from build123d import *

# Parameters (mm, degrees)
F1_DEPTH  = 76.2
F2_R      = 12.7
F3_DEPTH  = 76.201
F5_DEPTH  = 152.401
F6_R      = 38.1
F7_R      = 15.875
F8_DEPTH  = 6.35
F11_DEPTH = 12.7
F13_SIZE  = 1.524


with BuildPart() as f1:
    # F0 (on Front) → F1 (new body, symmetric)
    with BuildSketch(Plane.XZ):
        Polygon((-76.2, 0), (0, 0), (0, 152.4), (-25.4, 152.4), (-25.4, 25.4), (-76.2, 25.4), align=None)
    extrude(amount=F1_DEPTH, both=True)

    # F2 (on face) → F3 (cut, through all)
    with BuildSketch(Plane.YZ):
        with Locations((0, 114.3)):
            Circle(F2_R)
    extrude(amount=-F3_DEPTH, mode=Mode.SUBTRACT)

    # F4 (on face) → F5 (cut, through all)
    with BuildSketch(Plane(origin=(0, 0, 0), x_dir=(1, 0, 0), z_dir=(0, 0, -1))):
        with BuildLine():
            Line((-76.2, 12.7), (-76.2, -12.7))
            Line((-76.2, -12.7), (-63.5, -12.7))
            ThreePointArc((-63.5, -12.7), (-50.8, 0), (-63.5, 12.7))
            Line((-63.5, 12.7), (-76.2, 12.7))
        make_face()
    extrude(amount=-F5_DEPTH, mode=Mode.SUBTRACT)

    # F6
    f6_edges = [f1.edges().sort_by_distance(p)[0] for p in [
        (-12.7, 76.2, 152.4),
        (-12.7, -76.2, 152.4),
    ]]
    fillet(f6_edges, radius=F6_R)

    # F7 (on face) → F8 (cut)
    with BuildSketch(Plane(origin=(-25.4, 0, 0), x_dir=(0, -1, 0), z_dir=(-1, 0, 0))):
        with Locations((0, 114.3)):
            Circle(F7_R)
    extrude(amount=-F8_DEPTH, mode=Mode.SUBTRACT)

    # F10 (on offset) → F11 (join)
    with BuildSketch(Plane.XZ.offset(31.75)):
        Polygon((-25.4, 101.6), (-50.8, 25.4), (-25.4, 25.4), align=None)
    extrude(amount=F11_DEPTH)

    # F12: F1 across plane


with BuildPart() as f1_1:
    add(f1.part)
    add(f1.part.mirror(Plane.XZ))

    # F13
    f13_edges = [f1_1.edges().sort_by_distance(p)[0] for p in [
        (-25.4, 15.875, 114.3),
        (-19.05, -12.7, 114.3),
    ]]
    chamfer(f13_edges, length=F13_SIZE)


solid = f1_1.part
CAD build for the part. Positions are in the model's coordinates, mm. A direction names the side the tool comes from. Round coordinates to 2 decimals unless told otherwise and drop trailing zeros. Loops run counter-clockwise (first coordinate to the right, second up) from the corner with the lowest first, then second, coordinate; pieces in that order, holes last. Notation, with made-up numbers: M 16.25,59.25 L 54.25,59.25 A29 cw 54.25,91.25 Z; hole C 76,58 d10. An arc over 180 degrees is marked long. One line per question, with ' | ' between items. Start each with the question number.
Item 1: Wall check: line 1 (Y direction, x = -69, z = 22.5); line 2 (Z direction, x = -12, y = 0); line 3 (Y direction, x = -29, z = 79). Give the ranges that are in metal, low to high.
Item 2: Two-plate mould, pull along Z, no slides. Class faces 5 (the cylindrical face through (-8.64, -2.75, 101.9)), 6 (the flat face through (-37.922, 38.011, 64.033)), 7 (the flat face through (-39, -1, 0)), 8 (the flat face through (-22, -76.2, 45)): pulls with the +Z half, pulls with the -Z half, needs draft (parallel to the pull), parting line crosses it, or undercut.
Item 3: Which spindle directions (+Z, -Z, +X, -X, +Y, -Y) get a long thin tool onto all of the face, cutting with end or side? Do faces 1 (the flat face through (-33, -31.75, 47)), 2 (the flat face through (-19.05, 11, 124)), 3 (the flat face through (-70, 12.7, 13)), 4 (the flat face through (-33, 44.45, 47)). Say none if no direction does.
Item 4: Cut at D-D, the plane x = -39.5. Write the cut outline in (y, z).
Item 5: Cut at A-A, the plane y = 0. Write the cut outline in (x, z) (3 decimals).
Item 6: Cut at C-C, the plane z = 83. Write the cut outline in (x, y), plus the area to 3 significant figures.
Item 7: Pin check, flat tips, straight feed: pin 1 Ø10 at (y, z) = (0, 30.5) entering from -X; pin 2 Ø4 at (x, z) = (-21, 130) entering from +Y; pin 3 Ø4 at (x, z) = (-49, 41) entering from -Y; pin 4 Ø7.5 at (x, z) = (-35, 50) entering from -Y. Stop position of each tip, or through.
Item 8: Cut at B-B, the plane x = -61. Write the cut outline in (y, z), plus the area to 3 significant figures.
Responses:
1) line 1: y = -76.2 to -12.7, 12.7 to 76.2 | line 2: z = 0 to 101.6, 127 to 152.4 | line 3: y = -44.45 to -31.75, 31.75 to 44.45
2) face 5: undercut | face 6: pulls with the +Z half | face 7: pulls with the -Z half | face 8: needs draft
3) face 1: +Z, -X | face 2: -X | face 3: +Z, -Z, -X | face 4: +Z, -X, +Y
4) outline: M -76.2,0 L 76.2,0 L 76.2,25.4 L 44.45,25.4 L 44.45,59.3 L 31.75,59.3 L 31.75,25.4 L -31.75,25.4 L -31.75,59.3 L -44.45,59.3 L -44.45,25.4 L -76.2,25.4 Z
5) outline: M -50.8,0 L 0,0 L 0,101.6 L -17.526,101.6 L -19.05,100.076 L -19.05,98.425 L -23.876,98.425 L -25.4,96.901 L -25.4,25.4 L -50.8,25.4 Z; M -25.4,131.699 L -23.876,130.175 L -19.05,130.175 L -19.05,128.524 L -17.526,127 L 0,127 L 0,152.4 L -25.4,152.4 Z
6) outline: M -31.6,-44.45 L -25.4,-44.45 L -25.4,-76.2 L 0,-76.2 L 0,76.2 L -25.4,76.2 L -25.4,44.45 L -31.6,44.45 L -31.6,31.75 L -25.4,31.75 L -25.4,-31.75 L -31.6,-31.75 Z | area: 4,030 mm²
7) pin 1: stops at x = -25.4 | pin 2: stops at y = 73.65 | pin 3: passes through | pin 4: stops at y = -44.45
8) outline: M -76.2,0 L -12.45,0 L -12.45,25.4 L -76.2,25.4 Z; M 12.45,0 L 76.2,0 L 76.2,25.4 L 12.45,25.4 Z | area: 3,240 mm²
